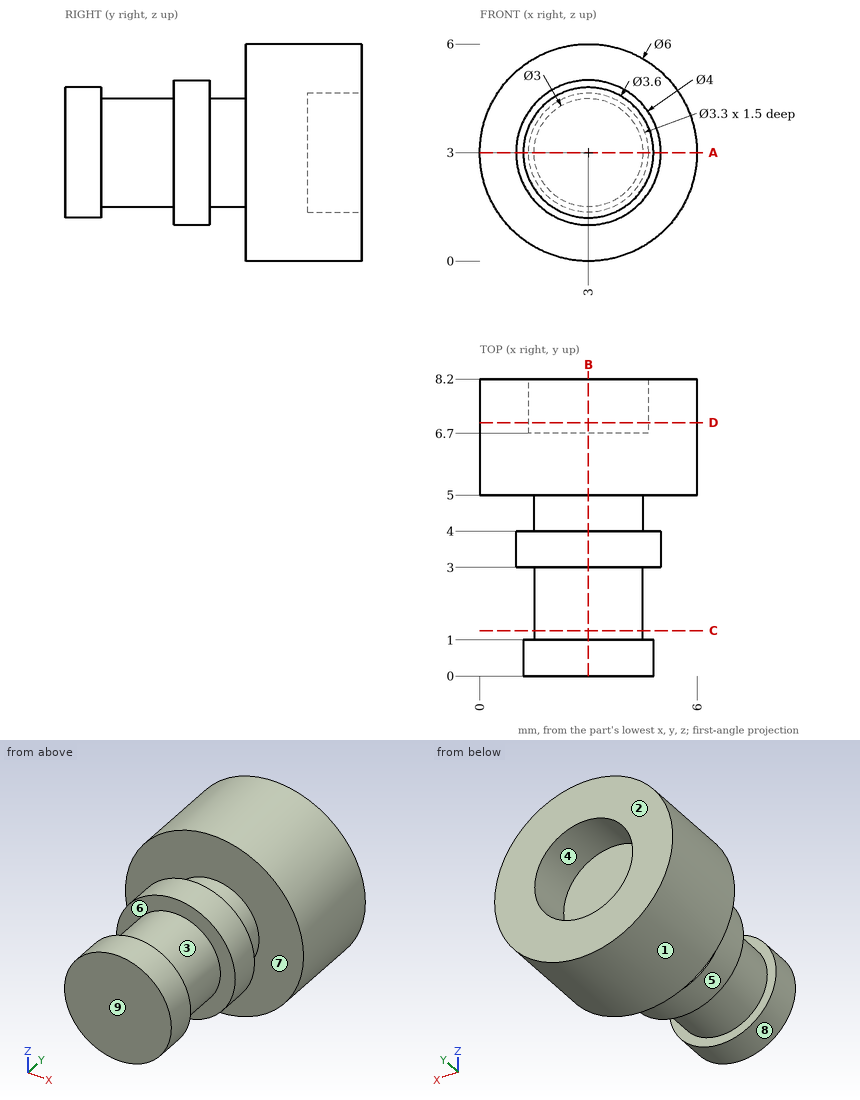
Here's the drawing with two shaded views (mm, measured from the low corner). I have some questions. A direction names the side the tool comes from. Give positions to 0.01 mm unless a question says otherwise; leave off trailing zeros. Loops run counter-clockwise (first coordinate to the right, second up) from the corner with the lowest first, then second, coordinate; pieces in that order, holes last. Notation, with made-up numbers: (-7.75, 74) -> (19.25, 74) arc R12 cw to (19.25, 89) -> close; hole circle Ø5 at (42.25, 49.5). An arc over 180 degrees is marked (long way). Use one line per item in the form item = value.
1) If we section it at C-C (y = 1.25): Please give me the cut outline in (x, z).
Answers:
outline = circle Ø3 at (3, 3)
2) If we section it at B-B (x = 3): Please give me the cut outline in (y, z).
Answers:
outline = (0, 1.2) -> (1, 1.2) -> (1, 1.5) -> (3, 1.5) -> (3, 1) -> (4, 1) -> (4, 1.5) -> (5, 1.5) -> (5, 0) -> (8.2, 0) -> (8.2, 1.35) -> (6.7, 1.35) -> (6.7, 4.65) -> (8.2, 4.65) -> (8.2, 6) -> (5, 6) -> (5, 4.5) -> (4, 4.5) -> (4, 5) -> (3, 5) -> (3, 4.5) -> (1, 4.5) -> (1, 4.8) -> (0, 4.8) -> close
3) If we section it at D-D (y = 7): Please give me the cut outline in (x, z).
Answers:
outline = circle Ø6 at (3, 3); hole circle Ø3.3 at (3, 3)
4) Will this pin go through, and if not, where does the flat tip stop? pin 1 (1.2 mm diameter, centred on x = 2.5, z = 2.5, fed in from +Y).
Answers:
pin_1 = 6.7
5) We'd pull the mould along Y, two halves only. Please class the marked faces 6, 7, 8 and 9: released by +Y, released by -Y, zero draft, split by the parting line, or undercut.
Answers:
face_6 = undercut
face_7 = undercut
face_8 = zero draft
face_9 = released by -Y
6) For the marked faces 1, 2, 3, 4 and 5, which set-ups out of +Z, -Z, +X, -X, +Y, -Y let a thin tool reach every point of the face, with its end or its side?
Answers:
face_1 = +Y, -Y
face_2 = +Z, -Z, +X, -X, +Y
face_3 = none
face_4 = +Y
face_5 = -Y
7) I need wall thicknesses on line 1 along Y through (x, z) = (3.85, 4.5); line 2 along X through (y, z) = (7.35, 3). Which ranges of each line are inside material? Lowest first, please.
Answers:
line_1 = 0 to 1, 3 to 4, 5 to 8.2
line_2 = 0 to 1.35, 4.65 to 6
8) If we section it at A-A (z = 3): Please give me the cut outline in (x, y).
Answers:
outline = (0, 5) -> (1.5, 5) -> (1.5, 4) -> (1, 4) -> (1, 3) -> (1.5, 3) -> (1.5, 1) -> (1.2, 1) -> (1.2, 0) -> (4.8, 0) -> (4.8, 1) -> (4.5, 1) -> (4.5, 3) -> (5, 3) -> (5, 4) -> (4.5, 4) -> (4.5, 5) -> (6, 5) -> (6, 8.2) -> (4.65, 8.2) -> (4.65, 6.7) -> (1.35, 6.7) -> (1.35, 8.2) -> (0, 8.2) -> close
